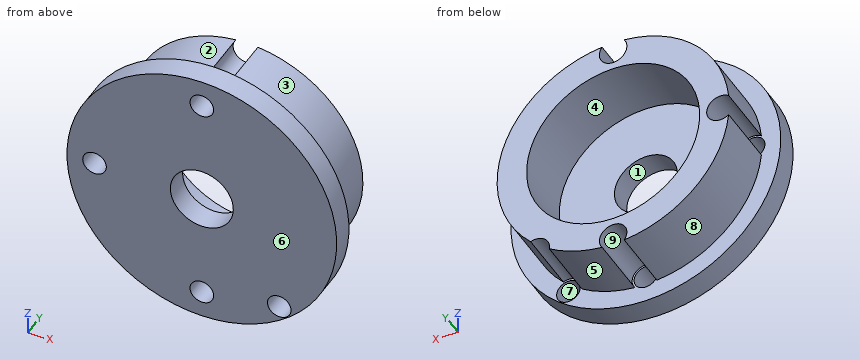
from build123d import *

# Parameters (mm, degrees)
CROQUIS2_R                   = 1.5
CORTAR_EXTRUIR1_DEPTH        = 10
CROQUIS3_R                   = 1.5
SALIENTE_EXTRUIR1_DEPTH      = 3
CROQUIS4_R                   = 1.5
CORTAR_EXTRUIR2_DEPTH        = 10
SALIENTE_EXTRUIR2_DEPTH      = 4
SALIENTE_EXTRUIR2_DEPTH_BACK = 4
CROQUIS5_R                   = 14.75
CROQUIS5_R_2                 = 11.75
CORTAR_EXTRUIR3_START        = -12
CROQUIS6_R                   = 1.5
CORTAR_EXTRUIR3_DEPTH        = 12
CROQUIS8_R                   = 10.142857143
CORTAR_EXTRUIR4_DEPTH        = 9
CROQUIS9_R                   = 1.75
CORTAR_EXTRUIR6_DEPTH        = 8
CROQUIS10_R                  = 11.75
CROQUIS10_R_2                = 11.125
SALIENTE_EXTRUIR3_DEPTH      = 10
CROQUIS11_R                  = 11.125
CROQUIS11_R_2                = 11
SALIENTE_EXTRUIR4_DEPTH      = 10


with BuildPart() as part:
    # Croquis1 → Revolución1 (revolve)
    with BuildSketch(Plane.XY, mode=Mode.PRIVATE) as revoluci_n1_sk:
        Polygon((-4, 0), (-4, 7), (-5, 7), (-10.142857143, 3), (-17.142857143, 3), (-17.142857143, 0), (-14, 0), align=None)
    revolve(revoluci_n1_sk.sketch.rotate(Axis((0, 0, 0), (0, 1, 0)), 270), axis=Axis((0, 0, 0), (0, 1, 0)))

    # Croquis2 → Cortar-Extruir1 (cut)
    with BuildSketch(Plane(origin=(0, 3, 0), x_dir=(1, 0, 0), z_dir=(0, 1, 0))):
        with Locations(Location((0, 13.64, 0), (0, 0, 270))):
            Circle(CROQUIS2_R)
        with Locations(Location((13.64, 0, 0), (0, 0, 270))):
            Circle(CROQUIS2_R)
        with Locations(Location((0, -13.64, 0), (0, 0, 270))):
            Circle(CROQUIS2_R)
        with Locations(Location((-13.64, 0, 0), (0, 0, 270))):
            Circle(CROQUIS2_R)
    extrude(amount=-CORTAR_EXTRUIR1_DEPTH, mode=Mode.SUBTRACT)

    # Croquis3 → Saliente-Extruir1 (add)
    with BuildSketch(Plane(origin=(0, 3, 0), x_dir=(1, 0, 0), z_dir=(0, 1, 0))):
        with Locations((13.64, 0)):
            Circle(CROQUIS3_R)
    extrude(amount=-SALIENTE_EXTRUIR1_DEPTH)

    # Croquis4 → Cortar-Extruir2 (cut)
    with BuildSketch(Plane(origin=(0, 0, 0), x_dir=(-1, 0, 0), z_dir=(0, -1, 0))):
        with Locations(Location((-9.844736786, 11.997981397, 0), (0, 0, 90))):
            Circle(CROQUIS4_R)
    extrude(amount=-CORTAR_EXTRUIR2_DEPTH, mode=Mode.SUBTRACT)

    # Croquis5 → Saliente-Extruir2 (add, two sides: drawn at the far end of the back side and taken through both)
    with BuildSketch(Plane(origin=(0, 7, 0), x_dir=(1, 0, 0), z_dir=(0, 1, 0)).offset(-SALIENTE_EXTRUIR2_DEPTH_BACK)):
        with Locations(Location((0, 0, 0), (0, 0, 85.923723928))):
            Circle(CROQUIS5_R)
        with Locations(Location((0, 0, 0), (0, 0, 270))):
            Circle(CROQUIS5_R_2, mode=Mode.SUBTRACT)
    extrude(amount=SALIENTE_EXTRUIR2_DEPTH + SALIENTE_EXTRUIR2_DEPTH_BACK)

    # Croquis6 → Cortar-Extruir3 (cut)
    with BuildSketch(Plane(origin=(0, 0, 0), x_dir=(-1, 0, 0), z_dir=(0, -1, 0)).offset(CORTAR_EXTRUIR3_START)):
        with Locations(Location((13.64, 0, 0), (0, 0, 270))):
            Circle(CROQUIS6_R)
        with Locations(Location((0, -13.64, 0), (0, 0, 270))):
            Circle(CROQUIS6_R)
        with Locations(Location((-9.844736786, 11.997981397, 0), (0, 0, 90))):
            Circle(CROQUIS6_R)
        with Locations(Location((0, 13.64, 0), (0, 0, 270))):
            Circle(CROQUIS6_R)
    extrude(amount=CORTAR_EXTRUIR3_DEPTH, mode=Mode.SUBTRACT)

    # Croquis8 → Cortar-Extruir4 (cut)
    with BuildSketch(Plane(origin=(0, 3, 0), x_dir=(1, 0, 0), z_dir=(0, 1, 0))):
        Circle(CROQUIS8_R)
    extrude(amount=CORTAR_EXTRUIR4_DEPTH, mode=Mode.SUBTRACT)

    # Croquis9 → Cortar-Extruir6 (cut)
    with BuildSketch(Plane(origin=(0, 11, 0), x_dir=(1, 0, 0), z_dir=(0, 1, 0))):
        with Locations((9.844736786, 11.997981397)):
            Circle(CROQUIS9_R)
        with Locations((0, 13.64)):
            Circle(CROQUIS9_R)
        with Locations((-13.64, 0)):
            Circle(CROQUIS9_R)
        with Locations((0, -13.64)):
            Circle(CROQUIS9_R)
    extrude(amount=-CORTAR_EXTRUIR6_DEPTH, mode=Mode.SUBTRACT)

    # Croquis10 → Saliente-Extruir3 (add)
    with BuildSketch(Plane(origin=(0, 11, 0), x_dir=(1, 0, 0), z_dir=(0, 1, 0))):
        Circle(CROQUIS10_R)
        with Locations(Location((0, 0, 0), (0, 0, 270))):
            Circle(CROQUIS10_R_2, mode=Mode.SUBTRACT)
    extrude(amount=-SALIENTE_EXTRUIR3_DEPTH)

    # Croquis11 → Saliente-Extruir4 (add)
    with BuildSketch(Plane(origin=(0, 11, 0), x_dir=(1, 0, 0), z_dir=(0, 1, 0))):
        Circle(CROQUIS11_R)
        with Locations(Location((0, 0, 0), (0, 0, 270))):
            Circle(CROQUIS11_R_2, mode=Mode.SUBTRACT)
    extrude(amount=-SALIENTE_EXTRUIR4_DEPTH)


solid = part.part
Input: part model. Units: mm. Frame: model coordinates. Face numbers are marked on the shaded views. A direction names the side the tool comes from. Give positions to 0.01 mm unless a question says otherwise; leave off trailing zeros. Write each loop counter-clockwise with the first axis right and the second up, starting at its lowest first coordinate (ties: lowest second). Pieces come first, ordered by that corner, then holes.
Q1. Material intervals for probe 1 along X at (y, z) = (1, 0); probe 2 along X at (y, z) = (6.5, 0); probe 3 along X at (y, z) = (2, 15), sorted ascending.
Q2. Section B-B, the plane y = 9. Output: boundary loops of the cut face in (x, z), plus the area to 3 significant figures.
Q3. Set-up query: the marked faces 5, 6, 7, 8 and 9. Return all of +Z, -Z, +X, -X, +Y, -Y with unobstructed straight access to the full face (end or side cutting, diameter ignored); none if empty.
Q4. Section A-A, the plane z = 0. Output: boundary loops of the cut face in (x, y), plus the area to 3 significant figures.
Q5. Pull-direction query (Z, two-part tool) for the marked faces 1, 2, 3 and 4; classes: pulls with the +Z half, pulls with the -Z half, needs draft (parallel to the pull), parting line crosses it, or undercut.
Q6. First-contact query: P1, Ø4, axis at x = 0, z = -13.64, coming from the +Y side; P2, Ø5, axis at x = -11, y = 1.5, coming from the +Z side; P3, Ø6, axis at x = -4.5, z = -6.5, coming from the +Y side; P4, Ø7, axis at x = 0, z = 0, coming from the +Y side. Flat tips, straight axial feed; report the tip coordinate or a pass-through.
Q7. Section D-D, the plane x = -13.64. Output: boundary loops of the cut face in (y, z).
Q8. Section C-C, the plane x = 0. Output: boundary loops of the cut face in (y, z), plus the area to 3 significant figures.
Filled in:
1. probe 1: x = -17.14 to -15.14, -12.14 to -4, 4 to 17.14
1. probe 2: x = -11.89 to -11, 11 to 14.75
1. probe 3: x = -8.3 to -0.63, 0.63 to 8.3
2. outline: (-14.68, -1.41) arc R14.75 ccw to (-1.41, -14.68) arc R1.75 cw (long way) to (1.41, -14.68) arc R14.75 ccw to (8.12, -12.31) arc R1.75 cw to (10.49, -10.37) arc R14.75 ccw to (1.41, 14.68) arc R1.75 cw (long way) to (-1.41, 14.68) arc R14.75 ccw to (-14.68, 1.41) arc R1.75 cw (long way) to start; hole circle Ø22 at (0, 0)
2. area: 276 mm2
3. face 5: -Z, +X, +Y
3. face 6: +Z, -Z, +X, -X, -Y
3. face 7: +Y, -Y
3. face 8: -Z, -X, +Y
3. face 9: +Y
4. outline: (-17.14, 0) - (-15.14, 0) - (-15.14, 3) - (-17.14, 3) - close; (-12.14, 0) - (-4, 0) - (-4, 3) - (-11, 3) - (-11, 11) - (-11.89, 11) - (-11.89, 3) - (-12.14, 3) - close; (4, 0) - (17.14, 0) - (17.14, 3) - (14.75, 3) - (14.75, 11) - (11, 11) - (11, 3) - (4, 3) - close
4. area: 107 mm2
5. face 1: undercut
5. face 2: pulls with the +Z half
5. face 3: parting line crosses it
5. face 4: undercut
6. P1: stops at y = 11
6. P2: stops at z = 14.89
6. P3: stops at y = 3
6. P4: passes through
7. outline: (0, -10.38) - (3, -10.38) - (3, -5.61) - (11, -5.61) - (11, -1.75) - (3, -1.75) - (3, -1.5) - (0, -1.5) - close; (0, 1.5) - (3, 1.5) - (3, 1.75) - (11, 1.75) - (11, 5.61) - (3, 5.61) - (3, 10.38) - (0, 10.38) - close
8. outline: (0, -17.14) - (3, -17.14) - (3, -15.14) - (0, -15.14) - close; (0, -12.14) - (3, -12.14) - (3, -11.89) - (11, -11.89) - (11, -11) - (3, -11) - (3, -4) - (0, -4) - close; (0, 4) - (3, 4) - (3, 11) - (11, 11) - (11, 11.89) - (3, 11.89) - (3, 12.14) - (0, 12.14) - close; (0, 15.14) - (3, 15.14) - (3, 17.14) - (0, 17.14) - close
8. area: 75.1 mm2
